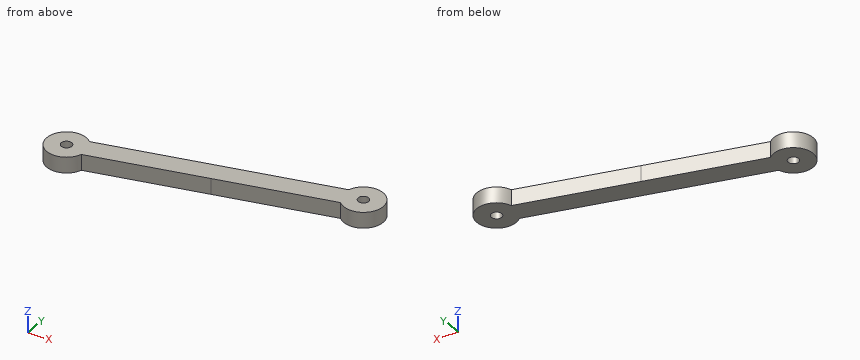
from build123d import *

# Parameters (mm, degrees)
SKETCH1_R           = 7.5
SKETCH1_R_2         = 3
SKETCH1_R_3         = 2
BOSS_EXTRUDE1_DEPTH = 6


with BuildPart() as part:
    # Sketch1 → Boss-Extrude1 (new body)
    # profile 1 of 4: a face of its own
    with BuildSketch(Plane(origin=(-250.576496127, -2880.89736156, 0), x_dir=(0.2387018630194584, 0.9710929000827057, 0), z_dir=(0, 0, 1))):
        with Locations((-56.392361751, 96.67944955)):
            Circle(SKETCH1_R)
        with Locations((-56.392361751, 96.67944955)):
            Circle(SKETCH1_R_2, mode=Mode.SUBTRACT)
    # profile 2 of 4: a face of its own
    with BuildSketch(Plane(origin=(-250.576496127, -2880.89736156, 0), x_dir=(0.2387018630194584, 0.9710929000827057, 0), z_dir=(0, 0, 1))):
        with BuildLine():
            ThreePointArc((-56.970497395, 89.201765471), (-52.893311506, 90.045698923), (-49.894496726, 92.934085733))
            Line((-49.894496726, 92.934085733), (-56.970497395, 89.201765471))
        make_face()
    # profile 3 of 4: a face of its own
    with BuildSketch(Plane(origin=(-250.576496127, -2880.89736156, 0), x_dir=(0.2387018630194584, 0.9710929000827057, 0), z_dir=(0, 0, 1))):
        with BuildLine():
            Line((-29.52735978, 54.320605501), (-49.894496726, 92.934085733))
            ThreePointArc((-49.894496726, 92.934085733), (-52.893311506, 90.045698923), (-56.970497395, 89.201765471))
            Line((-56.970497395, 89.201765471), (-36.603360449, 50.588285239))
            Line((-36.603360449, 50.588285239), (-29.52735978, 54.320605501))
        make_face()
    # profile 4 of 4: a face of its own
    with BuildSketch(Plane(origin=(-250.576496127, -2880.89736156, 0), x_dir=(0.2387018630194584, 0.9710929000827057, 0), z_dir=(0, 0, 1))):
        with Locations((-56.392361751, 96.67944955)):
            Circle(SKETCH1_R_2)
        with Locations(Location((-56.392361751, 96.67944955, 0), (0, 0, 283.809935935))):
            Circle(SKETCH1_R_3, mode=Mode.SUBTRACT)
    extrude(amount=BOSS_EXTRUDE1_DEPTH)

    # Mirror3: part across plane


with BuildPart() as part_1:
    add(part.part)
    add(part.part.mirror(Plane(origin=(-972.146788094, -242.383417146, 6), x_dir=(0, 0, 1), z_dir=(-0.9702957262759991, -0.2419218955996574, 0))))


solid = part_1.part
Check sheet for the modelled part. Datum: model origin and axes. Units: mm. Give positions to 0.01 mm unless a question says otherwise; leave off trailing zeros. Loops run counter-clockwise (first coordinate to the right, second up) from the corner with the lowest first, then second, coordinate; pieces in that order, holes last. Notation, with made-up numbers: M -1,-9.75 L 4,-9.75 A30 ccw 4,24.25 Z; hole C 29,31.25 d1. An arc over 180 degrees is marked long. Return JSON: item names as keys, results as strings. Group by question number.
1. Go/stop test with flat-tipped pins: pin 1 (3 mm diameter, centred on x = -269.5, z = 5.5, fed in from -Y); pin 2 (3 mm diameter, centred on x = -325.5, y = -2902, fed in from -Z); pin 3 (1 mm diameter, centred on y = -2908, z = 3.5, fed in from -X). Record where each tip stops, or that it passes through.
2. Cross-section at A-A on z = 2.9. Record the boundary of the cut face in (x, y).
3. Cross-section at B-B on x = -285.5. Record the boundary of the cut face in (y, z).
4. Cross-section at C-C on y = -2901.5. Record the boundary of the cut face in (x, z).
5. Thickness scan on L1, parallel to Y at x = -358.5, z = 2.25; L2, parallel to X at y = -2886, z = 0.6; L3, parallel to Y at x = -354, z = 3.1. Record the ranges inside material, lowest first.
Return value:
{
 "1": {"pin 1": "y = -2895.03", "pin 2": "z = 0", "pin 3": "x = -364.21"},
 "2": {"outline": "M -352.73,-2907.17 A7.5 ccw long -350.8,-2914.93 L -266.08,-2893.81 A7.5 ccw long -268.02,-2886.04 Z; hole C -357.92,-2912.58 d4; hole C -260.89,-2888.39 d4"},
 "3": {"outline": "M -2898.65,0 L -2890.4,0 L -2890.4,6 L -2898.65,6 Z"},
 "4": {"outline": "M -330.01,0 L -296.94,0 L -296.94,6 L -330.01,6 Z"},
 "5": {"L1": "-2920.06 to -2914.5, -2910.67 to -2905.1", "L2": "-268 to -253.78", "L3": "-2918.97 to -2906.19"}
}
